Verification items for the finished model (mm, model axes). A direction names the side the tool comes from. Give positions to 0.01 mm unless a question says otherwise; leave off trailing zeros. Order: outer loops, then holes, each group sorted by start corner. A loop starts at its lowest first (then second) coordinate and runs counter-clockwise, first axis right, second up. Notation, with made-up numbers: (-16, 49.5) -> (23, 49.5) arc R22 cw to (23, 75.5) -> close; hole circle Ø6 at (-26.75, 27). An arc over 180 degrees is marked (long way). Return JSON: item names as keys, results as strings. Group by question number.
(1) Cross-section at B-B on x = 18. Enter the section's corners in (y, z).
(2) Release check for a two-part mould opening along Z. For faces 4 (the face through (25, 10, 0)), 5 (the face through (-20.5, 10, 0.1)), 6 (the face through (17, 10, 10)) record: pulls with the +Z half, pulls with the -Z half, needs draft (parallel to the pull), parting line crosses it, or undercut.
(3) Cross-section at D-D on z = 11. Enter the section's corners in (x, y), then the cut area to 3 significant figures.
(4) Cross-section at C-C on y = 9.6. Enter the section's corners in (x, z), then the cut area to 3 significant figures.
(5) Thickness scan on line 1 along X through (y, z) = (10.65, 0); line 2 along Z through (x, y) = (-18, 10.1); line 3 along Z through (x, y) = (-14.5, 9.9). Record the ranges inside material, lowest first.
(6) Cross-section at A-A on z = 0. Enter the section's corners in (x, y).
(7) Tool access check on faces 1 (the face through (9, 10, 15)), 2 (the face through (-17, 10, 10)), 3 (the face through (0, 10, -10)). Record the directions out of +Z, -Z, +X, -X, +Y, -Y that give a thin tool (end or side, any length) a straight path to the whole face; none if there is none.
(8) Depth check by flat-ended pin: pin 1 Ø12 at (x, z) = (-10, 11) entering from +Y; pin 2 Ø1 at (y, z) = (9.5, 13.5) entering from +X; pin 3 Ø4.5 at (x, z) = (-18, 0) entering from +Y. Enter the tip coordinate at first touch or a pass-through.
Autodesk Inventor part; units mm, degrees
ref_plane "Work Plane1" through (-25, 9, -10) normal (0, 1, 0) x (1, 0, 0)
ref_plane "YZ Plane" through (0, 0, 0) normal (1, 0, 0) x (0, 1, 0)
ref_plane "XZ Plane" through (0, 0, 0) normal (0, 1, 0) x (-1, 0, 0)
ref_plane "Work Plane1" through (-25, 9, -10) normal (0, 1, 0) x (1, 0, 0)
sketch "Sketch1" plane through (-25, 9, -10) normal (0, 1, 0) x (1, 0, 0)
  line L0 (0, 0) -> (0, -20)
  line L1 (50, -20) -> (50, 0)
  line L2 (0, 0) -> (50, 0)
  line L3 (50, 0) -> (50, -20)
  line L4 (50, -20) -> (0, -20)
  line L5 (0, -20) -> (0, 0)
  line L6 (34, -20) -> (34, -30)
  line L7 (16, -30) -> (34, -30)
  line L8 (34, -20) -> (16, -20)
  line L9 (16, -20) -> (16, -30)
  line L10 (16, -30) -> (34, -30)
  line L11 (34, -30) -> (34, -20)
  circle A0 centre (7, -10) radius 2.5
  circle A1 centre (7, -10) radius 2.5
  circle A2 centre (43, -10) radius 2.5
  circle A3 centre (43, -10) radius 2.5
  point P0 (25, -10)
extrude "Extrusion1" add sketch "Sketch1" along normal blind 2
properties part number "gps_lid"
Verdict:
{
 "1": {"outline": "(9, -10) -> (11, -10) -> (11, -2.5) -> (9, -2.5) -> close; (9, 2.5) -> (11, 2.5) -> (11, 10) -> (9, 10) -> close"},
 "2": {"face 4": "needs draft", "face 5": "undercut", "face 6": "pulls with the +Z half"},
 "3": {"outline": "(-9, 9) -> (9, 9) -> (9, 11) -> (-9, 11) -> close", "area": "36.0 mm²"},
 "4": {"outline": "(-25, -10) -> (25, -10) -> (25, 10) -> (9, 10) -> (9, 20) -> (-9, 20) -> (-9, 10) -> (-25, 10) -> close; hole circle Ø5 at (-18, 0); hole circle Ø5 at (18, 0)", "area": "1,140 mm²"},
 "5": {"line 1": "-25 to -20.5, -15.5 to 15.5, 20.5 to 25", "line 2": "-10 to -2.5, 2.5 to 10", "line 3": "-10 to 10"},
 "6": {"outline": "(-25, 9) -> (-20.5, 9) -> (-20.5, 11) -> (-25, 11) -> close; (-15.5, 9) -> (15.5, 9) -> (15.5, 11) -> (-15.5, 11) -> close; (20.5, 9) -> (25, 9) -> (25, 11) -> (20.5, 11) -> close"},
 "7": {"face 1": "+Z, +X, +Y, -Y", "face 2": "+Z, -X, +Y, -Y", "face 3": "-Z, +X, -X, +Y, -Y"},
 "8": {"pin 1": "y = 11", "pin 2": "x = 9", "pin 3": "through"}
}
